Autodesk Inventor part; units mm, degrees
ref_plane "YZ Plane" through (0, 0, 0) normal (1, 0, 0) x (0, 1, 0)
ref_plane "XZ Plane" through (0, 0, 0) normal (0, 1, 0) x (-1, 0, 0)
ref_plane "XY Plane" through (0, 0, 0) normal (0, 0, 1) x (1, 0, 0)
sketch "Sketch1" plane through (0, 0, 0) normal (0, 1, 0) x (-1, 0, 0)
  arc A0 (-0.611111, -10.983012) -> (-0.611111, 10.983012) centre (0, 0) ccw
  line L0 (0, 0) -> (-108, 0) construction
  arc A1 (-108.277778, 4.992278) -> (-108.277778, -4.992278) centre (-108, 0) ccw
  line L1 (-0.611111, 10.983012) -> (-108.277778, 4.992278)
  line L2 (-0.611111, -10.983012) -> (-108.277778, -4.992278)
  circle A2 centre (0, 0) radius 6
  line L3 (-108.222222, 3.993822) -> (-0.555556, 9.984556)
  arc A3 (-0.555556, -9.984556) -> (-0.555556, 9.984556) centre (0, 0) ccw
  line L4 (-0.555556, -9.984556) -> (-108.222222, -3.993822)
  arc A4 (-108.222222, 3.993822) -> (-108.222222, -3.993822) centre (-108, 0) ccw
  line L5 (-95, -4.729527) -> (-95, 4.729527)
  point P0 (-100, 0)
  dimension "d0" = 22
  dimension "d1" = 108
  dimension "d2" = 10
  dimension "d3" = 8
  dimension "d6" = 12
  dimension "d7" = 1
  dimension "d8" = 13
extrude "Extrusion1" add sketch "Sketch1" against normal blind 3 contours L2 A1 L1 A0 | A2 | L3 L5 L4 A4 | L3 A3 L4 L5
sketch "Sketch1 outline for Extrusion2" plane through (0, 0, 0) normal (0, 1, 0) x (-1, 0, 0)
  arc A0 (-0.555556, -9.984556) -> (-0.555556, 9.984556) centre (0, 0) ccw
  line L0 (-95, -4.729527) -> (-0.555556, -9.984556)
  line L1 (-95, 4.729527) -> (-95, -4.729527)
  line L2 (-0.555556, 9.984556) -> (-95, 4.729527)
extrude "Extrusion2" add sketch "Sketch1 outline for Extrusion2" along normal blind 3 draft -20
extrude "Extrusion3" add sketch "Sketch1" against normal blind 5 contours A2
hole "Hole1" at (108, 0, 0) at (100, 0, 0) direction (0, -1, 0) diameter 2.8 end through all
hole "Hole2" at (0, -5, 0) direction (0, 1, 0) diameter 3.5 end through all
hole "Hole3" at (0, -5, 0) direction (0, 1, 0) diameter 8 depth 5
properties part number "servo arm TGY-S8166M long"
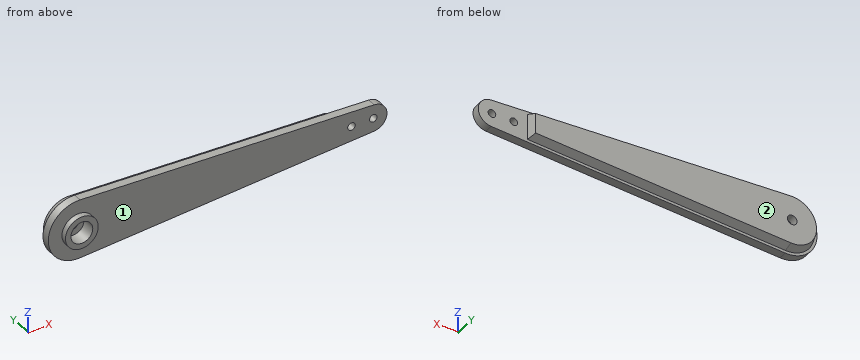
CAD build for the part. Positions are in the model's coordinates, mm. Face numbers are marked on the shaded views. Coordinates: 2 decimals unless noted, no trailing zeros. Order: outer loops, then holes, each group sorted by start corner. A loop starts at its lowest first (then second) coordinate and runs counter-clockwise, first axis right, second up. Notation, with made-up numbers: (-8.75, -17.75) - (22.25, -17.75) arc R22 cw to (22.25, -3.75) - close; hole circle Ø8 at (-10.5, 19.25). An arc over 180 degrees is marked (long way). Answer in a Markdown table with one row per item.
1. Slice it at C-C, the plane x = 84. List the corners of the cut face in (y, z).
Answer:
| item | result |
|---|---|
| outline | (-3, -6.34) - (0, -6.34) - (0, -5.34) - (3, -4.25) - (3, 4.25) - (0, 5.34) - (0, 6.34) - (-3, 6.34) - close |
2. Slice it at D-D, the plane y = 1.5. List the corners of the cut face in (x, z), then the cut area to 3 significant figures.
Answer:
| item | result |
|---|---|
| outline | (0.53, -9.44) - (94.45, -4.21) - (94.45, 4.21) - (0.53, 9.44) arc R9.45 ccw (long way) to start; hole circle Ø3.5 at (0, 0) |
| area | 1,420 mm² |
3. Drill centre lines: L1, parallel to X at y = -2.3, z = 0; L2, parallel to Z at x = 0, y = -3.7; L3, parallel to X at y = -1.25, z = -1.25. Where is each one in solid material? Low to high. Write a range as from..to.
Answer:
| item | result |
|---|---|
| L1 | -11..-4, 4..98.6, 101.4..106.6, 109.4..113 |
| L2 | -6..-4, 4..6 |
| L3 | -10.93..-3.8, 3.8..99.37, 100.63..107.37, 108.63..112.84 |
4. Slice it at B-B, the plane x = 100. List the corners of the cut face in (y, z), then the cut area to 3 significant figures.
Answer:
| item | result |
|---|---|
| outline | (-3, -5.45) - (0, -5.45) - (0, -1.4) - (-3, -1.4) - close; (-3, 1.4) - (0, 1.4) - (0, 5.45) - (-3, 5.45) - close |
| area | 24.3 mm² |
5. Flat gauge pins, fed straight in: P1, Ø2.5, axis at x = 1, z = -1.5, coming from the -Y side; P2, Ø1, axis at y = 0, z = -3, coming from the -X side; P3, Ø1, axis at x = 46, y = 0, coming from the -Z side. Where does each tip first touch, or does it go through?
Answer:
| item | result |
|---|---|
| P1 | y = 0 |
| P2 | x = -10.71 |
| P3 | z = -8.49 |
6. Slice it at A-A, the plane z = 0. List the corners of the cut face in (x, y), then the cut area to 3 significant figures.
Answer:
| item | result |
|---|---|
| outline | (-11, -3) - (-6, -3) - (-6, -5) - (-4, -5) - (-4, 0) - (-1.75, 0) - (-1.75, 3) - (-8.91, 3) - (-10, 0) - (-11, 0) - close; (1.75, 0) - (4, 0) - (4, -5) - (6, -5) - (6, -3) - (98.6, -3) - (98.6, 0) - (95, 0) - (93.91, 3) - (1.75, 3) - close; (101.4, -3) - (106.6, -3) - (106.6, 0) - (101.4, 0) - close; (109.4, -3) - (113, -3) - (113, 0) - (109.4, 0) - close |
| area | 640 mm² |
7. Pull direction Y, two halves, no side cores. Call the marked faces 1 and 2: +Y half, -Y half, draft (parallel to the pull), parting line (faces both ways), or undercut.
Answer:
| item | result |
|---|---|
| face 1 | -Y half |
| face 2 | +Y half |
